from build123d import *

# Parameters (mm, degrees)
SKETCH1_W           = 48.26
SKETCH1_H           = 17.78
BOSS_EXTRUDE1_DEPTH = 15.24
CUT_EXTRUDE1_DEPTH  = 7.62
CUT_EXTRUDE2_DEPTH  = 18.78


with BuildPart() as part:
    # Sketch1 → Boss-Extrude1 (new body)
    with BuildSketch(Plane.XY):
        with Locations((24.13, 8.89)):
            Rectangle(SKETCH1_W, SKETCH1_H)
    extrude(amount=-BOSS_EXTRUDE1_DEPTH)

    # Sketch3 → Cut-Extrude1 (cut)
    with BuildSketch(Plane(origin=(0, 17.78, 0), x_dir=(1, 0, 0), z_dir=(0, 1, 0))):
        Polygon((48.26, 15.24), (40.64, 7.62), (48.26, 0), align=None)
    extrude(amount=-CUT_EXTRUDE1_DEPTH, mode=Mode.SUBTRACT)

    # Sketch4 → Cut-Extrude2 (cut, through all)
    with BuildSketch(Plane(origin=(0, 17.78, 0), x_dir=(1, 0, 0), z_dir=(0, 1, 0))):
        with BuildLine():
            Line((34.83, 5.62), (27.21, 5.62))
            ThreePointArc((27.21, 5.62), (25.21, 7.62), (27.21, 9.62))
            Line((27.21, 9.62), (34.83, 9.62))
            ThreePointArc((34.83, 9.62), (36.83, 7.62), (34.83, 5.62))
        make_face()
        with BuildLine():
            Line((18.13, 5.62), (10.51, 5.62))
            ThreePointArc((10.51, 5.62), (8.51, 7.62), (10.51, 9.62))
            Line((10.51, 9.62), (18.13, 9.62))
            ThreePointArc((18.13, 9.62), (20.13, 7.62), (18.13, 5.62))
        make_face()
    extrude(amount=-CUT_EXTRUDE2_DEPTH, mode=Mode.SUBTRACT)


solid = part.part
Can you work these out from the model? Positions are in its coordinate system, mm. A direction names the side the tool comes from. Coordinates: 2 decimals unless noted, no trailing zeros. Order: outer loops, then holes, each group sorted by start corner. A loop starts at its lowest first (then second) coordinate and runs counter-clockwise, first axis right, second up. Notation, with made-up numbers: (-21, -31.5) -> (-16, -31.5) arc R6 cw to (-16, -20.5) -> close; hole circle Ø10 at (30.5, 9.5). An arc over 180 degrees is marked (long way). Use one line per item in the form item = value.
Q1. Imagine slicing it at A-A, the plane y = 11.5. List the corners of the cut face in (x, z) for me.
From the geometry:
outline = (0, -15.24) -> (48.26, -15.24) -> (40.64, -7.62) -> (48.26, 0) -> (0, 0) -> close; hole (10.51, -9.62) -> (18.13, -9.62) arc R2 ccw to (18.13, -5.62) -> (10.51, -5.62) arc R2 ccw to start; hole (27.21, -9.62) -> (34.83, -9.62) arc R2 ccw to (34.83, -5.62) -> (27.21, -5.62) arc R2 ccw to start
Q2. I need wall thicknesses on L1, parallel to Z at x = 27.5, y = 15.25; L2, parallel to X at y = 9.75, z = -8; L3, parallel to X at y = 13.75, z = -7.25. Which ranges of each line are inside material? Lowest first, please.
From the geometry:
L1 = -15.24 to -9.62, -5.62 to 0
L2 = 0 to 8.55, 20.09 to 25.25, 36.79 to 48.26
L3 = 0 to 8.54, 20.1 to 25.24, 36.8 to 41.01
Q3. Imagine slicing it at C-C, the plane z = -1.75. List the corners of the cut face in (x, y) for me, then the cut area to 3 significant figures.
From the geometry:
outline = (0, 0) -> (48.26, 0) -> (48.26, 10.16) -> (46.51, 10.16) -> (46.51, 17.78) -> (0, 17.78) -> close
area = 845 mm²
Q4. We'd pull the mould along X, two halves only. Please class faces 4 (the face through (0, 9, -8)), 5 (the face through (20.13, 9.01, -7.66)), 6 (the face through (44.5, 14.02, -11.48)): released by +X, released by -X, zero draft, split by the parting line, or undercut.
From the geometry:
face_4 = released by -X
face_5 = undercut
face_6 = released by +X
Q5. Which directions (+Z, -Z, +X, -X, +Y, -Y) give clear straight access to the entire face, cutting with the end or side of a thin tool? Please do faces 1 (the face through (36.83, 9.01, -7.66)), 2 (the face through (24, 9, 0)), 3 (the face through (45, 10.16, -8)).
From the geometry:
face_1 = +Y, -Y
face_2 = +Z, +X, -X, +Y, -Y
face_3 = +X, +Y
Q6. Imagine slicing it at B-B, the plane z = -10.25. List the corners of the cut face in (x, y) for me.
From the geometry:
outline = (0, 0) -> (48.26, 0) -> (48.26, 10.16) -> (43.27, 10.16) -> (43.27, 17.78) -> (0, 17.78) -> close
